from build123d import *

# Parameters (mm, degrees)
SKETCH1_R               = 3.75
SKETCH1_R_2             = 2.5
BOSS_EXTRUDE1_DEPTH     = 2.5
SKETCH2_R               = 2.150581317
BOSS_EXTRUDE2_DEPTH     = 5.5
CUT_EXTRUDE1_DEPTH      = 5.5
CUT_EXTRUDE1_DEPTH_BACK = 5.5
SKETCH5_R               = 1
BOSS_EXTRUDE4_DEPTH     = 5.5


with BuildPart() as part:
    # Sketch1 → Boss-Extrude1 (new body)
    with BuildSketch(Plane(origin=(0, 0, 0), x_dir=(1, 0, 0), z_dir=(0, 1, 0))):
        Circle(SKETCH1_R)
        Circle(SKETCH1_R_2, mode=Mode.SUBTRACT)
        with BuildLine():
            Line((0, -5.75), (0, -3.75))
            ThreePointArc((0, -3.75), (-2.105774565, -3.102936268), (-3.484844943, -1.385047191))
            Line((-3.484844943, -1.385047191), (-1.75, -5.75))
            Line((-1.75, -5.75), (0, -5.75))
        make_face()
        with BuildLine():
            ThreePointArc((3.484844943, -1.385047191), (2.105774565, -3.102936268), (0, -3.75))
            Line((0, -3.75), (0, -5.75))
            Line((0, -5.75), (1.75, -5.75))
            Line((1.75, -5.75), (3.484844943, -1.385047191))
        make_face()
    extrude(amount=BOSS_EXTRUDE1_DEPTH)

    # Sketch2 → Boss-Extrude2 (add)
    with BuildSketch(Plane.XY.offset(5.75)):
        with Locations((0, 1.25)):
            Circle(SKETCH2_R)
    extrude(amount=BOSS_EXTRUDE2_DEPTH)

    # Sketch4 → Cut-Extrude1 (cut, two sides)
    with BuildSketch(Plane(origin=(0, 0, 0), x_dir=(0, 0, -1), z_dir=(1, 0, 0))) as cut_extrude1_sk:
        Polygon((-5.75, -0.900581317), (-9.75, -0.900581317), (-5.75, 0), align=None)
        Polygon((-5.75, 3.400581317), (-5.75, 2.5), (-9.75, 3.400581317), align=None)
    extrude(amount=CUT_EXTRUDE1_DEPTH, mode=Mode.SUBTRACT)
    extrude(cut_extrude1_sk.sketch, amount=-CUT_EXTRUDE1_DEPTH_BACK, mode=Mode.SUBTRACT)

    # Sketch5 → Boss-Extrude4 (add)
    with BuildSketch(Plane.XY.offset(11.25)):
        Polygon((2.150581317, 1.25), (1.075290658, 3.112458053), (-1.075290658, 3.112458053), (-2.150581317, 1.25), (-1.075290658, -0.612458053), (1.075290658, -0.612458053), align=None)
        with Locations((0, 1.25)):
            Circle(SKETCH5_R, mode=Mode.SUBTRACT)
    extrude(amount=BOSS_EXTRUDE4_DEPTH)


solid = part.part
Read the model definition and answer for the solid it produces. Units are mm, in the model's axes. A direction names the side the tool comes from. Round coordinates to 2 decimals unless told otherwise and drop trailing zeros. Order: outer loops, then holes, each group sorted by start corner. A loop starts at its lowest first (then second) coordinate and runs counter-clockwise, first axis right, second up.
1) For faces 5 (the face through (-2.63, 1.23, 3.54)), 6 (the face through (-2, 0, 2)), 7 (the face through (0, -0.612, 14)), 8 (the face through (-1.6, 0.3, 14)), 9 (the face through (1.6, 2.2, 14)), determine the directions among +Z, -Z, +X, -X, +Y, -Y from which every point of the face is accessible in a straight line to the end or side of a thin tool.
2) The part is cut by section B-B on x = 0. Write down the section's boundary in (y, z).
3) Flat-ended cylindrical pins translate along their axes: pin 1 (1.5 mm diameter, centred on y = 2.5, z = 6, fed in from -X); pin 2 (1.7 mm diameter, centred on x = 0.5, z = 13, fed in from +Y); pin 3 (3 mm diameter, centred on x = -1, z = 5.5, fed in from +Y); pin 4 (4 mm diameter, centred on x = 0, z = 0, fed in from -Y). Find the tip coordinate at first contact, or state that the pin passes through.
4) Straight lines are drawn through the part: L1, parallel to X at y = 1.3, z = 0; L2, parallel to Y at x = 0, z = 14.45; L3, parallel to Y at x = -0.75, z = 16. For each, find the intervals that lie inside material, in ascending order.
5) The part is cut by section C-C on z = 12. Write down the section's boundary in (x, y), plus the area to 3 significant figures.
6) The part is cut by section D-D on y = -0.2. Write down the section's boundary in (x, z).
7) The mould has two halves that part along X. Classify faces 1 (the face through (-0.217, 0.274, 13.962)), 2 (the face through (0, 1, 11.25)), 3 (the face through (-1.6, 2.2, 14)), 4 (the face through (0.1, 1.23, -3.75)): released by +X, released by -X, zero draft, split by the parting line, or undercut.
8) The part is cut by section A-A on z = 0. Write down the section's boundary in (x, y), plus the area to 3 significant figures.
Resolved:
1. face 5: -X, +Y, -Y
1. face 6: -Z, +X, -X, -Y
1. face 7: +Z, +X, -X, -Y
1. face 8: +Z, -X, -Y
1. face 9: +Z, +X, +Y
2. outline: (-0.9, 9.75) - (0, 5.75) - (0, 2.5) - (2.5, 2.5) - (2.5, 5.75) - (3.4, 9.75) - (3.4, 11.25) - (3.11, 11.25) - (3.11, 16.75) - (2.25, 16.75) - (2.25, 11.25) - (0.25, 11.25) - (0.25, 16.75) - (-0.61, 16.75) - (-0.61, 11.25) - (-0.9, 11.25) - close; (0, -3.75) - (2.5, -3.75) - (2.5, -2.5) - (0, -2.5) - close
3. pin 1: stops at x = -2.09
3. pin 2: stops at y = 3.11
3. pin 3: stops at y = 2.78
3. pin 4: passes through
4. L1: x = -3.75 to -2.5, 2.5 to 3.75
4. L2: y = -0.61 to 0.25, 2.25 to 3.11
4. L3: y = -0.61 to 0.59, 1.91 to 3.11
5. outline: (-2.15, 1.25) - (-1.08, -0.61) - (1.08, -0.61) - (2.15, 1.25) - (1.08, 3.11) - (-1.08, 3.11) - close; hole circle Ø2 at (0, 1.25)
5. area: 8.87 mm2
6. outline: (-1.59, 6.64) - (1.59, 6.64) - (1.59, 11.25) - (1.31, 11.25) - (1.31, 16.75) - (-1.31, 16.75) - (-1.31, 11.25) - (-1.59, 11.25) - close
7. face 1: undercut
7. face 2: undercut
7. face 3: released by -X
7. face 4: split by the parting line
8. outline: (-3.75, 0) - (-2.5, 0) - (-2.5, 2.5) - (-3.75, 2.5) - close; (2.5, 0) - (3.75, 0) - (3.75, 2.5) - (2.5, 2.5) - close
8. area: 6.25 mm2
